```python
from build123d import *

# Parameters (mm, degrees)
F1_W        = 180.8
F1_H        = 14.4
F1_W_2      = 174.8
F1_H_2      = 8.4
F2_DEPTH    = 24
F3_T1_DEPTH = 24
F5_DEPTH    = 4.35
F6_W        = 140.8
F6_H        = 14.4
F7_DEPTH    = 16
F8_R        = 5
F10_DEPTH   = 3


# Not quite as in the source:
# - a fillet or chamfer that OpenCascade refuses, or shapes differently, is made with other operations: its cross-section is extruded or revolved along the edge and cut away or added
# - a pattern or mirror of a feature is missing from the dataset's text; its kind, count and spacing are read off the source's solid


with BuildPart() as f2:
    # F1 (on Top) → F2 (new body)
    with BuildSketch(Plane.XY):
        Rectangle(F1_W, F1_H)
        Rectangle(F1_W_2, F1_H_2, mode=Mode.SUBTRACT)
    extrude(amount=F2_DEPTH)

    # F3: fillet of radius 2 on 4 edges, made by hand

    # F3_s2 → F3_t1 (join)
    with BuildSketch(Plane.XY):
        with BuildLine():
            ThreePointArc((87.4004, -2.1990343146), (86.8142135624, -3.6142135624), (85.3990343146, -4.2004))
            Line((85.3990343146, -4.2004), (85.3990343146, -4.4005365685))
            ThreePointArc((85.3990343146, -4.4005365685), (86.3995171573, -4.4001365685), (87.4, -4.4001365685))
            Line((87.4, -4.4001365685), (87.6001365685, -4.2))
            ThreePointArc((87.6001365685, -4.2), (87.6001365685, -3.1995171573), (87.6005365685, -2.1990343146))
            Line((87.6005365685, -2.1990343146), (87.4004, -2.1990343146))
        make_face()
        with BuildLine():
            ThreePointArc((87.4004, 2.1990343146), (86.8142135624, 3.6142135624), (85.3990343146, 4.2004))
            Line((85.3990343146, 4.2004), (85.3990343146, 4.4005365685))
            ThreePointArc((85.3990343146, 4.4005365685), (86.3995171573, 4.4001365685), (87.4, 4.4001365685))
            Line((87.4, 4.4001365685), (87.6001365685, 4.2))
            ThreePointArc((87.6001365685, 4.2), (87.6001365685, 3.1995171573), (87.6005365685, 2.1990343146))
            Line((87.6005365685, 2.1990343146), (87.4004, 2.1990343146))
        make_face()
        with BuildLine():
            ThreePointArc((-85.3990343146, -4.2004), (-86.8142135624, -3.6142135624), (-87.4004, -2.1990343146))
            Line((-87.4004, -2.1990343146), (-87.6005365685, -2.1990343146))
            ThreePointArc((-87.6005365685, -2.1990343146), (-87.6001365685, -3.1995171573), (-87.6001365685, -4.2))
            Line((-87.6001365685, -4.2), (-87.4, -4.4001365685))
            ThreePointArc((-87.4, -4.4001365685), (-86.3995171573, -4.4001365685), (-85.3990343146, -4.4005365685))
            Line((-85.3990343146, -4.4005365685), (-85.3990343146, -4.2004))
        make_face()
        with BuildLine():
            ThreePointArc((-87.4004, 2.1990343146), (-86.8142135624, 3.6142135624), (-85.3990343146, 4.2004))
            Line((-85.3990343146, 4.2004), (-85.3990343146, 4.4005365685))
            ThreePointArc((-85.3990343146, 4.4005365685), (-86.3995171573, 4.4001365685), (-87.4, 4.4001365685))
            Line((-87.4, 4.4001365685), (-87.6001365685, 4.2))
            ThreePointArc((-87.6001365685, 4.2), (-87.6001365685, 3.1995171573), (-87.6005365685, 2.1990343146))
            Line((-87.6005365685, 2.1990343146), (-87.4004, 2.1990343146))
        make_face()
    extrude(amount=F3_T1_DEPTH)

    # F4 (on Front) → F5 (join, symmetric)
    with BuildSketch(Plane.XZ):
        with BuildLine():
            ThreePointArc((87.4, 8.75), (85.0568542495, 3.0931457505), (79.4, 0.75))
            Line((79.4, 0.75), (79.4, 0))
            Line((79.4, 0), (90.4, 0))
            Line((90.4, 0), (90.4, 8.75))
            Line((90.4, 8.75), (87.4, 8.75))
        make_face()
    f5 = extrude(amount=F5_DEPTH, both=True)

    # F5_copies: F5 across plane
    add(f5.mirror(Plane(origin=(0, 0, 0), x_dir=(0, 0, -1), z_dir=(-1, 0, 0))))

    # F6 (on face) → F7 (cut)
    with BuildSketch(Plane.XY.offset(24)):
        Rectangle(F6_W, F6_H)
    extrude(amount=-F7_DEPTH, mode=Mode.SUBTRACT)

    # F8
    f8_edges = [f2.edges().sort_by_distance(p)[0] for p in [
        (-70.4, 5.7, 24),
        (-70.4, -5.7, 24),
        (70.4, 5.7, 24),
        (70.4, -5.7, 24),
    ]]
    fillet(f8_edges, radius=F8_R)

    # F9 (on Top) → F10 (join)
    with BuildSketch(Plane.XY):
        with BuildLine():
            Line((90.4, -7.2), (-90.4, -7.2))
            ThreePointArc((-90.4, -7.2), (0, -24.4878132379), (90.4, -7.2))
        make_face()
        with BuildLine():
            Line((-90.4, 7.2), (90.4, 7.2))
            ThreePointArc((90.4, 7.2), (0, 24.4878132379), (-90.4, 7.2))
        make_face()
    extrude(amount=F10_DEPTH)


solid = f2.part
```
Check sheet for the modelled part. Datum: model origin and axes. Units: mm. A direction names the side the tool comes from. Round coordinates to 2 decimals unless told otherwise and drop trailing zeros. Loops run counter-clockwise (first coordinate to the right, second up) from the corner with the lowest first, then second, coordinate; pieces in that order, holes last. Notation, with made-up numbers: (-3.75, 8.25) -> (50.25, 8.25) arc R6 ccw to (50.25, 17.25) -> close; hole circle Ø1 at (-37.5, 14.25). An arc over 180 degrees is marked (long way). Write item = value, one per line. Start each with the question number.
1) Set-up check for faces 1 (the cylindrical face through (85.119, -0.059, 3.156)), 2 (the flat face through (-70.4, 6, 14)), 3 (the flat face through (-88, 0, 24)): record each of +Z, -Z, +X, -X, +Y, -Y from which the full face is reachable in a straight line by a thin tool's end or side.
2) Sectioned sample at C-C, the plane x = 16. Record the cut outline in (y, z), plus the area to 3 significant figures.
3) Gauge pin test, flat ends, axial feed: pin 1 Ø1.5 at (x, y) = (-50.5, -18.5) entering from +Z; pin 2 Ø10.5 at (x, z) = (-18, 12.5) entering from +Y; pin 3 Ø12 at (x, z) = (30.5, 8.5) entering from +Y; pin 4 Ø1 at (x, y) = (21, 9) entering from -Z. Record the tip position at first contact, or that the pin passes through.
4) Thickness scan on probe 1 along X at (y, z) = (-1.5, 18); probe 2 along Y at (x, z) = (-75, 16.25); probe 3 along Y at (x, z) = (2, 2.5). Record the ranges inside material, lowest first.
5) Sectioned sample at B-B, the plane z = 10.5. Record the cut outline in (x, y).
6) Sectioned sample at A-A, the plane y = 0.5. Record the cut outline in (x, z).
7) Release check for a two-part mould opening along X. For faces 4 (the cylindrical face through (-1.296, -24.484, 1.479)), 5 (the flat face through (-1, -6, 8)), 6 (the flat face through (87.4, 0, 16)), 7 (the flat face through (-1, 14, 3)) record: released by +X, released by -X, zero draft, split by the parting line, or undercut.
8) Sectioned sample at D-D, the plane y = -11.5. Record the cut outline in (x, z), plus the area to 3 significant figures.
Results are:
q1.face_1 = +Z
q1.face_2 = +Z, +Y, -Y
q1.face_3 = +Z, +X, -X, +Y, -Y
q2.outline = (-23.96, 0) -> (-4.2, 0) -> (-4.2, 8) -> (-7.2, 8) -> (-7.2, 3) -> (-23.96, 3) -> close; (4.2, 0) -> (23.96, 0) -> (23.96, 3) -> (7.2, 3) -> (7.2, 8) -> (4.2, 8) -> close
q2.area = 149 mm^2
q3.pin_1 = 3
q3.pin_2 = 7.2
q3.pin_3 = 22.87
q3.pin_4 = 0
q4.probe_1 = -90.4 to -87.4, 87.4 to 90.4
q4.probe_2 = -7.2 to -4.2, 4.2 to 7.2
q4.probe_3 = -24.48 to -4.2, 4.2 to 24.48
q5.outline = (-90.4, -7.2) -> (-70.4, -7.2) -> (-70.4, -4.2) -> (-85.44, -4.2) arc R2 cw to (-87.4, -2.24) -> (-87.4, 2.24) arc R2 cw to (-85.44, 4.2) -> (-70.4, 4.2) -> (-70.4, 7.2) -> (-90.4, 7.2) -> close; (70.4, -7.2) -> (90.4, -7.2) -> (90.4, 7.2) -> (70.4, 7.2) -> (70.4, 4.2) -> (85.44, 4.2) arc R2 cw to (87.4, 2.24) -> (87.4, -2.24) arc R2 cw to (85.44, -4.2) -> (70.4, -4.2) -> close
q6.outline = (-90.4, 0) -> (-79.4, 0) -> (-79.4, 0.75) arc R8 cw to (-87.4, 8.75) -> (-87.4, 24) -> (-90.4, 24) -> close; (79.4, 0) -> (90.4, 0) -> (90.4, 24) -> (87.4, 24) -> (87.4, 8.75) arc R8 cw to (79.4, 0.75) -> close
q7.face_4 = split by the parting line
q7.face_5 = undercut
q7.face_6 = undercut
q7.face_7 = zero draft
q8.outline = (-78.71, 0) -> (78.71, 0) -> (78.71, 3) -> (-78.71, 3) -> close
q8.area = 472 mm^2
